Input: part model. Units: mm. Frame: model coordinates. Face numbers are marked on the shaded views. A direction names the side the tool comes from. Coordinates: 2 decimals unless noted, no trailing zeros. Write each loop counter-clockwise with the first axis right and the second up, starting at its lowest first coordinate (ties: lowest second). Pieces come first, ordered by that corner, then holes. Notation, with made-up numbers: (-37.75, 74.25) - (10.25, 74.25) arc R17 ccw to (10.25, 79.25) - close; hole circle Ø2 at (72, -7.75). An arc over 180 degrees is marked (long way). Put each result on its own line as item: value. Start each with the question number.
1. Cut plane C-C, the plane y = 1.85. Return loops of the section in (x, z), and give its area (3 significant figures).
2. Cut plane A-A, the plane z = 0. Return loops of the section in (x, y).
3. Line query: line 1 (Y direction, x = -4, z = 1.45); line 2 (Z direction, x = -0.5, y = 1.65); line 3 (Z direction, x = -3.5, y = 3.05). Output: solid intervals per line, ascending.
4. Pin query (flat end, axial travel): pin 1 (1.3 mm diameter, centred on x = -1, y = 2.5, fed in from +Z); pin 2 (1.3 mm diameter, centred on x = 0, y = 2.5, fed in from -Z); pin 3 (1 mm diameter, centred on y = 2, z = -1, fed in from +X). Return the tip coordinate at first contact, or that it passes through.
5. Cut plane B-B, the plane x = -0.5. Return loops of the section in (y, z), and give its area (3 significant figures).
6. Access query for the marked faces 1, 2, 3 and 4. Directions: +Z, -Z, +X, -X, +Y, -Y. A direction counts if a zero-diameter tool reaches every point of the face in a straight line with its end or side. Return the directions, or none.
from build123d import *

# Parameters (mm, degrees)
BOSS_EXTRUDE1_DEPTH = 0.7
BOSS_EXTRUDE2_DEPTH = 2.8
FILLET1_R           = 0.2
FILLET2_R           = 0.08
FILLET3_R           = 0.07


with BuildPart() as part:
    # Sketch1 → Boss-Extrude1 (new body)
    with BuildSketch(Plane(origin=(0, 0, 0), x_dir=(1, 0, 0), z_dir=(0, 1, 0))):
        with BuildLine():
            Line((-2.85, 2.2), (2.85, 2.2))
            ThreePointArc((2.85, 2.2), (5.05, 0), (2.85, -2.2))
            Line((2.85, -2.2), (-2.85, -2.2))
            ThreePointArc((-2.85, -2.2), (-5.05, 0), (-2.85, 2.2))
        make_face()
    extrude(amount=BOSS_EXTRUDE1_DEPTH)

    # Sketch2 → Boss-Extrude2 (add)
    with BuildSketch(Plane(origin=(0, 0.7, 0), x_dir=(1, 0, 0), z_dir=(0, 1, 0))):
        with BuildLine():
            Line((-2.85, 1.75), (2.85, 1.75))
            ThreePointArc((2.85, 1.75), (4.6, 0), (2.85, -1.75))
            Line((2.85, -1.75), (-2.85, -1.75))
            ThreePointArc((-2.85, -1.75), (-4.6, 0), (-2.85, 1.75))
        make_face()
    extrude(amount=BOSS_EXTRUDE2_DEPTH)

    # Fillet1
    fillet1_edges = [part.edges().sort_by_distance(p)[0] for p in [
        (-4.6, 3.5, 0),
        (0, 3.5, 1.75),
        (4.6, 3.5, 0),
        (0, 3.5, -1.75),
    ]]
    fillet(fillet1_edges, radius=FILLET1_R)

    # Fillet2
    fillet2_edges = [part.edges().sort_by_distance(p)[0] for p in [
        (5.05, 0.7, 0),
        (0, 0.7, -2.2),
        (-5.05, 0.7, 0),
        (0, 0, -2.2),
        (5.05, 0, 0),
        (0, 0, 2.2),
        (-5.05, 0, 0),
        (0, 0.7, 2.2),
    ]]
    fillet(fillet2_edges, radius=FILLET2_R)

    # Fillet3
    fillet3_edges = [part.edges().sort_by_distance(p)[0] for p in [
        (-4.6, 0.7, 0),
        (0, 0.7, 1.75),
        (4.6, 0.7, 0),
        (0, 0.7, -1.75),
    ]]
    fillet(fillet3_edges, radius=FILLET3_R)


solid = part.part
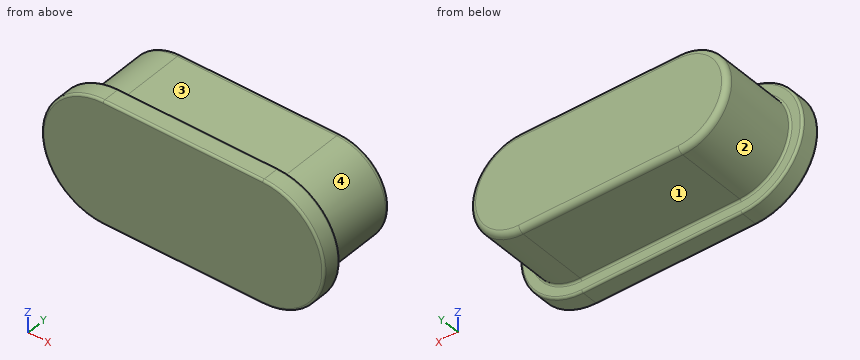
Report:
1. outline: (-2.85, -1.75) - (2.85, -1.75) arc R1.75 ccw to (2.85, 1.75) - (-2.85, 1.75) arc R1.75 ccw to start
1. area: 29.6 mm^2
2. outline: (-5.05, 0.08) arc R0.08 ccw to (-4.97, 0) - (4.97, 0) arc R0.08 ccw to (5.05, 0.08) - (5.05, 0.62) arc R0.08 ccw to (4.97, 0.7) - (4.67, 0.7) arc R0.07 cw to (4.6, 0.77) - (4.6, 3.3) arc R0.2 ccw to (4.4, 3.5) - (-4.4, 3.5) arc R0.2 ccw to (-4.6, 3.3) - (-4.6, 0.77) arc R0.07 cw to (-4.67, 0.7) - (-4.97, 0.7) arc R0.08 ccw to (-5.05, 0.62) - close
3. line 1: y = 0 to 0.7
3. line 2: z = -1.75 to 1.75
3. line 3: z = -1.62 to 1.62
4. pin 1: stops at z = 1.75
4. pin 2: stops at z = -1.75
4. pin 3: stops at x = 4.53
5. outline: (0, -2.12) arc R0.08 ccw to (0.08, -2.2) - (0.62, -2.2) arc R0.08 ccw to (0.7, -2.12) - (0.7, -1.82) arc R0.07 cw to (0.77, -1.75) - (3.3, -1.75) arc R0.2 ccw to (3.5, -1.55) - (3.5, 1.55) arc R0.2 ccw to (3.3, 1.75) - (0.77, 1.75) arc R0.07 cw to (0.7, 1.82) - (0.7, 2.12) arc R0.08 ccw to (0.62, 2.2) - (0.08, 2.2) arc R0.08 ccw to (0, 2.12) - close
5. area: 12.9 mm^2
6. face 1: -Z, +X, -X, +Y
6. face 2: -X, +Y
6. face 3: +Z, +X, -X, +Y
6. face 4: +X, +Y
